from build123d import *

# Parameters (mm, degrees)
F0_R     = 7.5
F1_DEPTH = 4
F2_R     = 5
F3_DEPTH = 7
F4_R     = 3.5
F5_DEPTH = 3
F6_SIZE  = 0.5


with BuildPart() as f1:
    # F0 (on Top) → F1 (new body)
    with BuildSketch(Plane.XY):
        Circle(F0_R)
    extrude(amount=F1_DEPTH)

    # F2 (on face) → F3 (join)
    with BuildSketch(Plane.XY.offset(4)):
        Circle(F2_R)
    extrude(amount=F3_DEPTH)

    # F4 (on face) → F5 (join)
    with BuildSketch(Plane.XY.offset(11)):
        Circle(F4_R)
    extrude(amount=F5_DEPTH)

    # F6
    f6_edges = [f1.edges().sort_by_distance(p)[0] for p in [
        (-3.5, 0, 14),
        (-5, 0, 11),
        (-7.5, 0, 4),
        (-7.5, 0, 0),
    ]]
    chamfer(f6_edges, length=F6_SIZE)


solid = f1.part
Model file for the job. Use its own axes, mm. A direction names the side the tool comes from. Coordinates: 2 decimals unless noted, no trailing zeros. Loops run counter-clockwise (first coordinate to the right, second up) from the corner with the lowest first, then second, coordinate; pieces in that order, holes last. Notation, with made-up numbers: (-7.75, 71) -> (6.25, 71) arc R16 cw to (6.25, 81) -> close; hole circle Ø10 at (-36.75, 54.25). An arc over 180 degrees is marked (long way). Use one line per item in the form item = value. Start each with the question number.
(1) Tool access for faces 1 (the flat face through (-5, 2, 4)), 2 (the cylindrical face through (-7.493, 0.33, 1.979)): list every direction of +Z, -Z, +X, -X, +Y, -Y with a clear straight run to the whole face (end or side of a thin tool).
(2) Cut at C-C on z = 6.75. Give the cut face in (x, y).
(3) Cut at A-A on x = 0. Give the cut face in (y, z).
(4) Probe probe 1 along Z at (x, y) = (4, 5); probe 2 along Z at (x, y) = (3.75, 0); probe 3 along Y at (x, z) = (0, 7). List the from-to ranges inside material, lowest first. Write a range as from..to.
(5) Flat gauge pins, fed straight in: pin 1 (6 mm diameter, centred on x = -5, z = 4.5, fed in from -Y); pin 2 (2 mm diameter, centred on y = -2, z = 4, fed in from +X); pin 3 (8 mm diameter, centred on y = 3.5, z = 10.5, fed in from +X). Where does each tip first touch, or does it go through?
Values:
q1.face_1 = +Z
q1.face_2 = +Z, -Z
q2.outline = circle Ø10 at (0, 0)
q3.outline = (-7.5, 0.5) -> (-7, 0) -> (7, 0) -> (7.5, 0.5) -> (7.5, 3.5) -> (7, 4) -> (5, 4) -> (5, 10.5) -> (4.5, 11) -> (3.5, 11) -> (3.5, 13.5) -> (3, 14) -> (-3, 14) -> (-3.5, 13.5) -> (-3.5, 11) -> (-4.5, 11) -> (-5, 10.5) -> (-5, 4) -> (-7, 4) -> (-7.5, 3.5) -> close
q4.probe_1 = 0..4
q4.probe_2 = 0..11
q4.probe_3 = -5..5
q5.pin_1 = -7.18
q5.pin_2 = 7.41
q5.pin_3 = 5
